from build123d import *

# Parameters (mm, degrees)
SKETCH2_W           = 160
SKETCH2_H           = 28.45
BOSS_EXTRUDE1_DEPTH = 10
SKETCH4_W           = 60
SKETCH4_H           = 10
BOSS_EXTRUDE2_DEPTH = 5
SKETCH5_R           = 2.5
CUT_EXTRUDE1_DEPTH  = 83.883053907


with BuildPart() as part:
    # Sketch2 → Boss-Extrude1 (new body)
    with BuildSketch(Plane(origin=(0, 0, 0), x_dir=(1, 0, 0), z_dir=(0, 1, 0))):
        Rectangle(SKETCH2_W, SKETCH2_H)
    extrude(amount=BOSS_EXTRUDE1_DEPTH)

    # Sketch4 → Boss-Extrude2 (add)
    with BuildSketch(Plane.XY.offset(14.225)):
        with Locations((0, 5)):
            Rectangle(SKETCH4_W, SKETCH4_H)
    extrude(amount=BOSS_EXTRUDE2_DEPTH)

    # Sketch5 → Cut-Extrude1 (cut, through all)
    with BuildSketch(Plane(origin=(0, 10, 0), x_dir=(1, 0, 0), z_dir=(0, 1, 0))):
        with Locations(Location((70, -6.225, 0), (0, 0, 270))):
            Circle(SKETCH5_R)
        with Locations(Location((30, -6.225, 0), (0, 0, 270))):
            Circle(SKETCH5_R)
        with Locations(Location((-30, -6.225, 0), (0, 0, 90))):
            Circle(SKETCH5_R)
        with Locations(Location((-70, -6.225, 0), (0, 0, 90))):
            Circle(SKETCH5_R)
    extrude(amount=-CUT_EXTRUDE1_DEPTH, mode=Mode.SUBTRACT)


solid = part.part
Can you work these out from the model? Positions are in its coordinate system, mm. A direction names the side the tool comes from. Coordinates: 2 decimals unless noted, no trailing zeros. Write each loop counter-clockwise with the first axis right and the second up, starting at its lowest first coordinate (ties: lowest second). Pieces come first, ordered by that corner, then holes.
Q1. Imagine slicing it at B-B, the plane x = 70. List the corners of the cut face in (y, z) for me (3 decimals).
Results found:
outline: (0, -14.225) - (10, -14.225) - (10, 3.725) - (0, 3.725) - close; (0, 8.725) - (10, 8.725) - (10, 14.225) - (0, 14.225) - close
Q2. If we mould it in two halves opening along Z, with no side actions, what happens to faces 4 (the face through (55, 5, 14.225)), 5 (the face through (-1, 10, 2)), 6 (the face through (67.56, 5.07, 5.68))? For each: +Z half, -Z half, draft (parallel to the pull), parting line (faces both ways), or undercut.
Results found:
face 4: +Z half
face 5: draft
face 6: undercut
Q3. Please list where these lines run through material, in increasing order: L1, parallel to X at y = 8.75, z = 6; L2, parallel to Z at x = -70, y = 7.5 (3 decimals); L3, parallel to X at y = 3.5, z = 5.
Results found:
L1: x = -80 to -72.49, -67.51 to -32.49, -27.51 to 27.51, 32.49 to 67.51, 72.49 to 80
L2: z = -14.225 to 3.725, 8.725 to 14.225
L3: x = -80 to -72.18, -67.82 to -32.18, -27.82 to 27.82, 32.18 to 67.82, 72.18 to 80
Q4. For P1, Ø4, axis at y = 2.5, z = 16.5, coming from the +X side; P2, Ø1.5, axis at y = 6.5, z = 15.5, coming from the -X side, each with a flat end and sliding along its axis, tell me the tip position at first contact or that it passes through.
Results found:
P1: stops at x = 30
P2: stops at x = -30
Q5. Which directions (+Z, -Z, +X, -X, +Y, -Y) give clear straight access to the entire face, cutting with the end or side of a thin tool? Please do faces 1 (the face through (-55, 5, 14.225)), 2 (the face through (31.69, 5.07, 4.382)), 3 (the face through (30, 5, 17)).
Results found:
face 1: +Z, -X, +Y, -Y
face 2: +Y, -Y
face 3: +Z, +X, +Y, -Y
Q6. Imagine slicing it at A-A, the plane y = 1.5. List the corners of the cut face in (x, z) for me (3 decimals).
Results found:
outline: (-80, -14.225) - (80, -14.225) - (80, 14.225) - (30, 14.225) - (30, 19.225) - (-30, 19.225) - (-30, 14.225) - (-80, 14.225) - close; hole circle Ø5 at (-70, 6.225); hole circle Ø5 at (-30, 6.225); hole circle Ø5 at (30, 6.225); hole circle Ø5 at (70, 6.225)
